Can you work these out from the drawing? Everything is in mm from the part's minimum corner. A direction names the side the tool comes from. Coordinates: 2 decimals unless noted, no trailing zeros. Write each loop counter-clockwise with the first axis right and the second up, starting at its lowest first coordinate (ties: lowest second). Pieces come first, ordered by that corner, then holes. Notation, with made-up numbers: (66.25, -33.5) - (73.25, -33.5) arc R15 ccw to (73.25, -20.5) - close; hole circle Ø2 at (32.25, 48). An arc over 180 degrees is marked (long way). One line per question, with ' | ' between items. Start each with the question number.
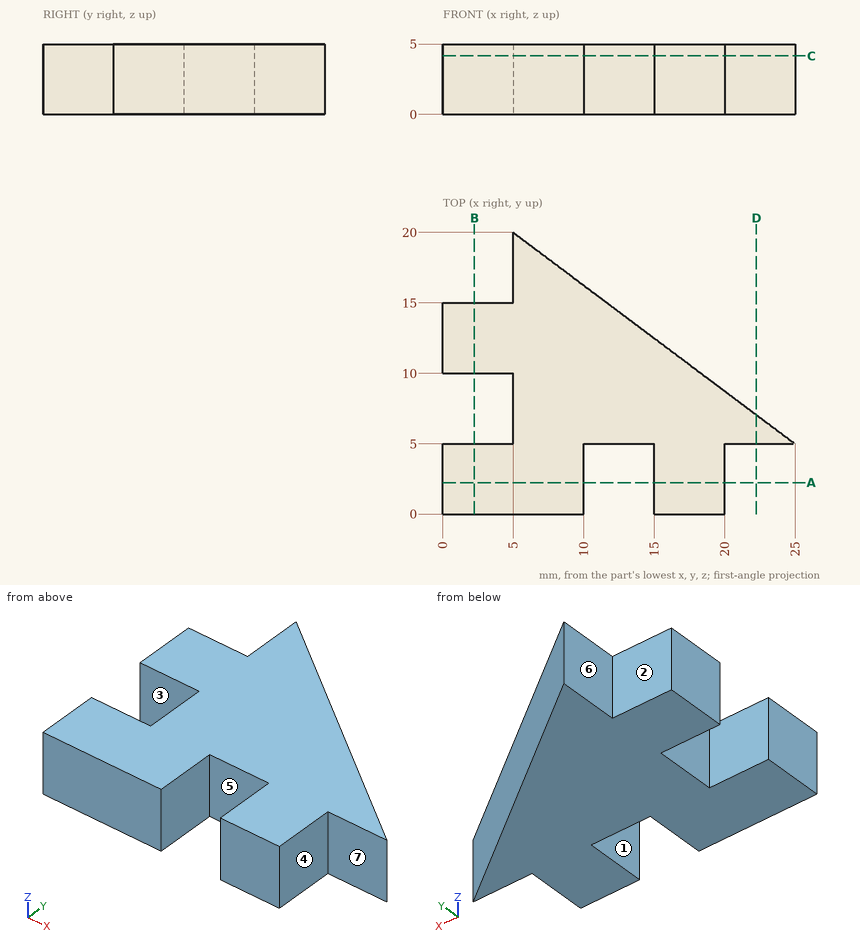
(1) If we section it at B-B on x = 2.25: List the corners of the cut face in (y, z) for me, plus the area to 3 significant figures.
(2) If we section it at C-C on z = 4.15: List the corners of the cut face in (x, y) for me.
(3) If we section it at A-A on y = 2.25: List the corners of the cut face in (x, z) for me.
(4) I'm going to push flat-ended pins straight in: pin 1 (3 mm diameter, centred on x = 17.5, z = 4.5, fed in from +Y); pin 2 (1 mm diameter, centred on x = 17, y = 13, fed in from -Z); pin 3 (2.5 mm diameter, centred on y = 3.5, z = 1.5, fed in from +X); pin 4 (1.5 mm diameter, centred on x = 23, z = 3, fed in from -Y). Where does each tip first touch, or does it pass through?
(5) If I drill on probe 1 along Y at (x, z) = (3.25, 0.95); probe 2 along X at (y, z) = (1.75, 3.85); probe 3 along X at (y, z) = (8.75, 4.6), over which ranges is the centre line in solid material (lowest first)?
(6) If we mould it in two halves opening along X, with no side actions, what happens to the marked faces 5, 6 and 7? For each: +X half, -X half, draft (parallel to the pull), parting line (faces both ways), or undercut.
(7) Which directions (+Z, -Z, +X, -X, +Y, -Y) give clear straight access to the entire face, cutting with the end or side of a thin tool? Please do the marked faces 1, 2, 3 and 4.
(8) If we section it at D-D on x = 22.25: List the corners of the cut face in (y, z) for me, plus the area to 3 significant figures.
Values:
1) outline: (0, 0) - (5, 0) - (5, 5) - (0, 5) - close; (10, 0) - (15, 0) - (15, 5) - (10, 5) - close | area: 50.0 mm2
2) outline: (0, 0) - (10, 0) - (10, 5) - (15, 5) - (15, 0) - (20, 0) - (20, 5) - (25, 5) - (5, 20) - (5, 15) - (0, 15) - (0, 10) - (5, 10) - (5, 5) - (0, 5) - close
3) outline: (0, 0) - (10, 0) - (10, 5) - (0, 5) - close; (15, 0) - (20, 0) - (20, 5) - (15, 5) - close
4) pin 1: y = 11.75 | pin 2: through | pin 3: x = 20 | pin 4: y = 5
5) probe 1: 0 to 5, 10 to 15 | probe 2: 0 to 10, 15 to 20 | probe 3: 5 to 20
6) face 5: undercut | face 6: -X half | face 7: draft
7) face 1: +Z, -Z, -Y | face 2: +Z, -Z, -X, +Y | face 3: +Z, -Z, -X | face 4: +Z, -Z, +X, -Y
8) outline: (5, 0) - (7.06, 0) - (7.06, 5) - (5, 5) - close | area: 10.3 mm2
